```python
from build123d import *

# Parameters (mm, degrees)
EXTRUDE_1_DEPTH = 2.1


with BuildPart() as part:
    # 草图1 → 凸台-拉伸1 (new body)
    with BuildSketch(Plane.XY):
        with BuildLine():
            Line((1.2, 0), (0, 0))
            Line((0, 0), (0, -2.4))
            ThreePointArc((0, -2.4), (0.74246212, -2.70753788), (1.05, -3.45))
            ThreePointArc((1.05, -3.45), (0.74246212, -4.19246212), (0, -4.5))
            Line((0, -4.5), (-2.1, -4.5))
            Line((-2.1, -4.5), (-2.1, -12.5))
            Line((-2.1, -12.5), (0, -12.5))
            ThreePointArc((0, -12.5), (0.74246212, -12.80753788), (1.05, -13.55))
            ThreePointArc((1.05, -13.55), (0.74246212, -14.29246212), (0, -14.6))
            Line((0, -14.6), (0, -17))
            Line((0, -17), (3, -17))
            Line((3, -17), (14.8, -3))
            Line((14.8, -3), (14.8, 0))
            Line((14.8, 0), (13.4, 0))
            ThreePointArc((13.4, 0), (12.35, -1.05), (11.3, 0))
            Line((11.3, 0), (11.3, 2.1))
            Line((11.3, 2.1), (3.3, 2.1))
            Line((3.3, 2.1), (3.3, 0))
            ThreePointArc((3.3, 0), (2.25, -1.05), (1.2, 0))
        make_face()
        Polygon((4, -11.158586353), (4, -4), (10.033665641, -4), align=None, mode=Mode.SUBTRACT)
    extrude(amount=EXTRUDE_1_DEPTH)


solid = part.part
```
The model under review builds one solid part; all positions refer to its coordinate system, in mm. A direction names the side the tool comes from. Round coordinates to 2 decimals unless told otherwise and drop trailing zeros. Loops run counter-clockwise (first coordinate to the right, second up) from the corner with the lowest first, then second, coordinate; pieces in that order, holes last.
1) Consider section A-A on z = 0.35. State the section outline as (x, y) points, then the cut area to 3 significant figures.
Values follow:
outline: (-2.1, -12.5) - (0, -12.5) arc R1.05 cw to (0, -14.6) - (0, -17) - (3, -17) - (14.8, -3) - (14.8, 0) - (13.4, 0) arc R1.05 cw to (11.3, 0) - (11.3, 2.1) - (3.3, 2.1) - (3.3, 0) arc R1.05 cw to (1.2, 0) - (0, 0) - (0, -2.4) arc R1.05 cw to (0, -4.5) - (-2.1, -4.5) - close; hole (4, -11.16) - (10.03, -4) - (4, -4) - close
area: 174 mm2
2) Consider section D-D on x = 0.5. State the section outline as (y, z) points.
Values follow:
outline: (-17, 0) - (-14.47, 0) - (-14.47, 2.1) - (-17, 2.1) - close; (-12.63, 0) - (-4.37, 0) - (-4.37, 2.1) - (-12.63, 2.1) - close; (-2.53, 0) - (0, 0) - (0, 2.1) - (-2.53, 2.1) - close
3) Tool access review of faces 1 (the face through (-1, -4.5, 1)), 2 (the face through (14, 0, 1)), 3 (the face through (2.27, -1.05, 1.04)), 4 (the face through (7.06, -7.53, 1.04)), 5 (the face through (-1, -12.5, 1)): name each direction out of +Z, -Z, +X, -X, +Y, -Y from which nothing blocks a thin tool from reaching the whole face with its end or side.
Values follow:
face 1: +Z, -Z, -X, +Y
face 2: +Z, -Z, +X, +Y
face 3: +Z, -Z, +Y
face 4: +Z, -Z
face 5: +Z, -Z, -X, -Y
4) The part is to be moulded in two halves that separate along X. For faces 6 (the face through (0, -16, 1)), 7 (the face through (7, 2.1, 1)), 8 (the face through (4, -8, 1)), say which applies: pulls with the +X half, pulls with the -X half, needs draft (parallel to the pull), parting line crosses it, or undercut.
Values follow:
face 6: pulls with the -X half
face 7: needs draft
face 8: undercut
5) Wall thickness on line 1 along Y through (x, z) = (0.25, 0.9); line 2 along Y through (x, z) = (-1.25, 0.1); line 3 along Y through (x, z) = (5, 0.4): over which ranges is each line inside the solid? List them lowest first.
Values follow:
line 1: y = -17 to -14.57, -12.53 to -4.47, -2.43 to 0
line 2: y = -12.5 to -4.5
line 3: y = -14.63 to -9.97, -4 to 2.1
6) Consider section B-B on x = 7.5. State the section outline as (y, z) points, then the cut area to 3 significant figures.
Values follow:
outline: (-11.66, 0) - (-7.01, 0) - (-7.01, 2.1) - (-11.66, 2.1) - close; (-4, 0) - (2.1, 0) - (2.1, 2.1) - (-4, 2.1) - close
area: 22.6 mm2
7) Consider section C-C on y = -4.25. State the section outline as (x, z) points.
Values follow:
outline: (0.68, 0) - (4, 0) - (4, 2.1) - (0.68, 2.1) - close; (9.82, 0) - (13.75, 0) - (13.75, 2.1) - (9.82, 2.1) - close
8) Clearance check with flat-ended pins moving along their axes: P1, Ø0.6, axis at x = 0.5, z = 1, coming from the +Y side; P2, Ø1, axis at y = -1, z = 1.5, coming from the -X side; P3, Ø1, axis at y = -6.5, z = 1.5, coming from the +X side. State where each tip first meets the part, or that it passes through.
Values follow:
P1: stops at y = 0
P2: stops at x = 0
P3: stops at x = 12.27
